```python
from build123d import *

# Parameters (mm, degrees)
F0_R     = 2.5
F0_R_2   = 0.5
F1_DEPTH = 5
F3_DEPTH = 5


with BuildPart() as f1:
    # F0 (on Top) → F1 (new body)
    with BuildSketch(Plane.XY):
        Circle(F0_R)
        Circle(F0_R_2, mode=Mode.SUBTRACT)
    extrude(amount=F1_DEPTH)

    # F2 (on Top) → F3 (join)
    with BuildSketch(Plane.XY):
        with BuildLine():
            ThreePointArc((-0.981539, 0.981539), (-0.933303, 1.027514), (-0.882916, 1.07112))
            Line((-0.882916, 1.07112), (-9.58502, 11.628184))
            Line((-9.58502, 11.628184), (-10.099932, 12.143096))
            Line((-10.099932, 12.143096), (-11.447009, 11.447009))
            Line((-11.447009, 11.447009), (-10.606602, 10.606602))
            Line((-10.606602, 10.606602), (-0.981539, 0.981539))
        make_face()
        with BuildLine():
            Line((0, 15), (0, 1.388106))
            ThreePointArc((0, 1.388106), (0.066617, 1.386507), (0.133081, 1.381712))
            Line((0.133081, 1.381712), (1.444735, 15))
            Line((1.444735, 15), (1.444735, 15.728196))
            Line((1.444735, 15.728196), (0, 16.188515))
            Line((0, 16.188515), (0, 15))
        make_face()
        with BuildLine():
            Line((10.606602, 10.606602), (0.981539, 0.981539))
            ThreePointArc((0.981539, 0.981539), (1.027514, 0.933303), (1.07112, 0.882916))
            Line((1.07112, 0.882916), (11.628184, 9.58502))
            Line((11.628184, 9.58502), (12.143096, 10.099932))
            Line((12.143096, 10.099932), (11.447009, 11.447009))
            Line((11.447009, 11.447009), (10.606602, 10.606602))
        make_face()
        with BuildLine():
            Line((15, 0), (1.388106, 0))
            ThreePointArc((1.388106, 0), (1.386507, -0.066617), (1.381712, -0.133081))
            Line((1.381712, -0.133081), (15, -1.444735))
            Line((15, -1.444735), (15.728196, -1.444735))
            Line((15.728196, -1.444735), (16.188515, 0))
            Line((16.188515, 0), (15, 0))
        make_face()
        with BuildLine():
            Line((10.606602, -10.606602), (0.981539, -0.981539))
            ThreePointArc((0.981539, -0.981539), (0.933303, -1.027514), (0.882916, -1.07112))
            Line((0.882916, -1.07112), (9.58502, -11.628184))
            Line((9.58502, -11.628184), (10.099932, -12.143096))
            Line((10.099932, -12.143096), (11.447009, -11.447009))
            Line((11.447009, -11.447009), (10.606602, -10.606602))
        make_face()
        with BuildLine():
            ThreePointArc((0, -1.388106), (-0.066617, -1.386507), (-0.133081, -1.381712))
            Line((-0.133081, -1.381712), (-1.444735, -15))
            Line((-1.444735, -15), (-1.444735, -15.728196))
            Line((-1.444735, -15.728196), (0, -16.188515))
            Line((0, -16.188515), (0, -15))
            Line((0, -15), (0, -1.388106))
        make_face()
        with BuildLine():
            ThreePointArc((-0.981539, -0.981539), (-1.027514, -0.933303), (-1.07112, -0.882916))
            Line((-1.07112, -0.882916), (-11.628184, -9.58502))
            Line((-11.628184, -9.58502), (-12.143096, -10.099932))
            Line((-12.143096, -10.099932), (-11.447009, -11.447009))
            Line((-11.447009, -11.447009), (-10.606602, -10.606602))
            Line((-10.606602, -10.606602), (-0.981539, -0.981539))
        make_face()
        with BuildLine():
            ThreePointArc((-1.388106, 0), (-1.386507, 0.066617), (-1.381712, 0.133081))
            Line((-1.381712, 0.133081), (-15, 1.444735))
            Line((-15, 1.444735), (-15.728196, 1.444735))
            Line((-15.728196, 1.444735), (-16.188515, 0))
            Line((-16.188515, 0), (-15, 0))
            Line((-15, 0), (-1.388106, 0))
        make_face()
    extrude(amount=F3_DEPTH)


solid = f1.part
```
Check sheet for the modelled part. Datum: model origin and axes. Units: mm. A direction names the side the tool comes from. Give positions to 0.01 mm unless a question says otherwise; leave off trailing zeros. Loops run counter-clockwise (first coordinate to the right, second up) from the corner with the lowest first, then second, coordinate; pieces in that order, holes last. Notation, with made-up numbers: M 7,5 L 17,5 A23 cw 17,24 Z; hole C -19,2 d6. An arc over 180 degrees is marked long. Answer in a Markdown table with one row per item.
1) Mould release check, pull along X, two halves, no side actions. Record for faces 1 (the face through (-7, -7, 2)), 2 (the face through (-1, -1, 0)), 3 (the face through (1.077, 2.256, 2.465)), 4 (the face through (-15.955, 0.732, 2.465)): released by +X, released by -X, zero draft, split by the parting line, or undercut.
Solutions:
| item | result |
|---|---|
| face 1 | undercut |
| face 2 | zero draft |
| face 3 | undercut |
| face 4 | released by -X |
2) Cross-section at B-B (x = 5). Enter the section's corners in (y, z), plus the area to 3 significant figures.
Solutions:
| item | result |
|---|---|
| outline | M -6.07,0 L -5,0 L -5,5 L -6.07,5 Z; M -0.48,0 L 0,0 L 0,5 L -0.48,5 Z; M 4.12,0 L 5,0 L 5,5 L 4.12,5 Z |
| area | 12.1 mm^2 |
3) Thickness scan on line 1 (Y direction, x = -9.5, z = 1.6) (3 decimals); line 2 (X direction, y = -9, z = 0.3); line 3 (Y direction, x = 11, z = 3.7). Record the ranges inside material, lowest first.
Solutions:
| item | result |
|---|---|
| line 1 | y = -9.5 to -7.831, 0 to 0.915, 9.5 to 11.525 |
| line 2 | x = -10.92 to -9, -0.87 to 0, 7.42 to 9 |
| line 3 | y = -11.68 to -11, -1.06 to 0, 9.07 to 11 |
4) Tool access check on faces 5 (the face through (-7, 7, 2)), 6 (the face through (2.256, -1.077, 2.465)), 7 (the face through (9, 0, 2)), 8 (the face through (7, 7, 2)). Record the directions out of +Z, -Z, +X, -X, +Y, -Y that give a thin tool (end or side, any length) a straight path to the whole face; none if there is none.
Solutions:
| item | result |
|---|---|
| face 5 | +Z, -Z, -X |
| face 6 | +Z, -Z |
| face 7 | +Z, -Z, +X |
| face 8 | +Z, -Z, +Y |
5) Depth check by flat-ended pin: pin 1 (0.6 mm diameter, centred on x = -15.5, z = 1.5, fed in from +Y); pin 2 (3 mm diameter, centred on y = -6, z = 1.5, fed in from -X); pin 3 (1.5 mm diameter, centred on x = -10.5, z = 2, fed in from -Y). Enter the tip coordinate at first touch or a pass-through.
Solutions:
| item | result |
|---|---|
| pin 1 | stops at y = 1.44 |
| pin 2 | stops at x = -9.1 |
| pin 3 | stops at y = -11.25 |
6) Cross-section at C-C (x = 13). Enter the section's corners in (y, z), plus the area to 3 significant figures.
Solutions:
| item | result |
|---|---|
| outline | M -1.25,0 L 0,0 L 0,5 L -1.25,5 Z |
| area | 6.26 mm^2 |
7) Cross-section at A-A (y = -8). Enter the section's corners in (x, z).
Solutions:
| item | result |
|---|---|
| outline | M -9.71,0 L -8,0 L -8,5 L -9.71,5 Z; M -0.77,0 L 0,0 L 0,5 L -0.77,5 Z; M 6.59,0 L 8,0 L 8,5 L 6.59,5 Z |
